Build history of the part. All positions in model axes, mm. Face numbers are marked on the shaded views. A direction names the side the tool comes from. Give positions to 0.01 mm unless a question says otherwise; leave off trailing zeros. Order: outer loops, then holes, each group sorted by start corner. A loop starts at its lowest first (then second) coordinate and runs counter-clockwise, first axis right, second up. Notation, with made-up numbers: M 31.5,-38 L 88.5,-38 A17 cw 88.5,-6 Z; hole C 9.5,55 d10. An arc over 180 degrees is marked long. Use CSV: the item, a comma, the result in double quotes. Start each with the question number.
Item 1: Wall check: line 1 along Z through (x, y) = (44, 17.75); line 2 along Z through (x, y) = (36.5, 1.25); line 3 along Y through (x, z) = (30.5, -3.5) (3 decimals). Give the ranges that are in metal, low to high.
Item 2: Band-saw the part on C-C on y = 22.5. Write the cut outline in (x, z), plus the area to 3 significant figures.
Item 3: Which spindle directions (+Z, -Z, +X, -X, +Y, -Y) get a long thin tool onto all of the face, cutting with end or side? Do the marked faces 1, 2 and 3. Say none if no direction does.
Item 4: Pin check, flat tips, straight feed: P1, Ø0.5, axis at x = 25, y = 1, coming from the -Z side; P2, Ø5, axis at x = 29, z = -4.5, coming from the -Y side (3 decimals); P3, Ø3, axis at x = 16.5, z = -2, coming from the +Y side (3 decimals); P4, Ø6, axis at y = 5.5, z = -3, coming from the -X side. Stop position of each tip, or through.
Item 5: Band-saw the part on B-B on z = -4. Write the cut outline in (x, y) (3 decimals), plus the area to 3 significant figures.
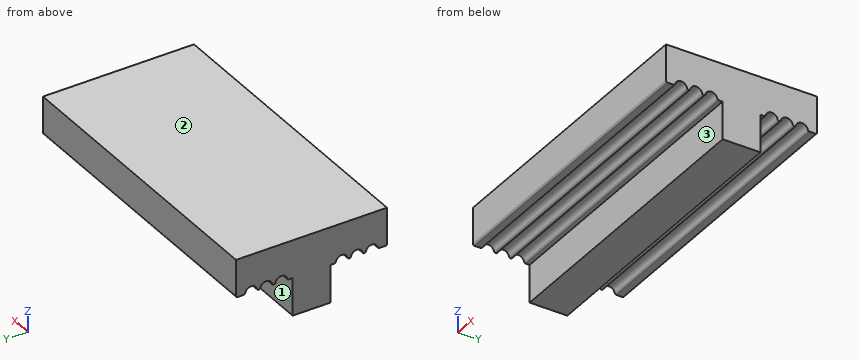
from build123d import *

# Parameters (mm, degrees)
F1_DEPTH = 50.8
F2_R     = 0.254


with BuildPart() as f1:
    # F0 (on Right) → F1 (new body)
    with BuildSketch(Plane.YZ):
        with BuildLine():
            Line((0, 6.35), (0, 0))
            Line((0, 0), (1.524, 0))
            ThreePointArc((1.524, 0), (2.54, 1.016), (3.556, 0))
            Line((3.556, 0), (4.064, 0))
            ThreePointArc((4.064, 0), (5.08, 1.016), (6.096, 0))
            Line((6.096, 0), (6.604, 0))
            ThreePointArc((6.604, 0), (7.62, 1.016), (8.636, 0))
            Line((8.636, 0), (9.525, 0))
            Line((9.525, 0), (9.525, -6.35))
            Line((9.525, -6.35), (15.875, -6.35))
            Line((15.875, -6.35), (15.875, 0))
            Line((15.875, 0), (16.764, 0))
            ThreePointArc((16.764, 0), (17.78, 1.016), (18.796, 0))
            Line((18.796, 0), (19.304, 0))
            ThreePointArc((19.304, 0), (20.32, 1.016), (21.336, 0))
            Line((21.336, 0), (21.844, 0))
            ThreePointArc((21.844, 0), (22.86, 1.016), (23.876, 0))
            Line((23.876, 0), (25.4, 0))
            Line((25.4, 0), (25.4, 6.35))
            Line((25.4, 6.35), (0, 6.35))
        make_face()
    extrude(amount=F1_DEPTH)

    # F2
    f2_edges = [f1.edges().sort_by_distance(p)[0] for p in [
        (25.4, 23.876, 0),
        (25.4, 25.4, 0),
        (25.4, 21.336, 0),
        (25.4, 18.796, 0),
        (25.4, 6.604, 0),
        (25.4, 4.064, 0),
        (25.4, 1.524, 0),
        (25.4, 0, 0),
        (25.4, 3.556, 0),
        (25.4, 6.096, 0),
        (25.4, 8.636, 0),
        (25.4, 16.764, 0),
        (25.4, 19.304, 0),
        (25.4, 21.844, 0),
    ]]
    fillet(f2_edges, radius=F2_R)


solid = f1.part
Model answer:
1,line 1,"z = 1.02 to 6.35"
1,line 2,"z = 0 to 6.35"
1,line 3,"y = 9.525 to 15.875"
2,outline,"M 0,0.95 L 50.8,0.95 L 50.8,6.35 L 0,6.35 Z"
2,area,"274 mm^2"
3,face 1,"-Z, +X, -X, +Y"
3,face 2,"+Z, +X, -X, +Y, -Y"
3,face 3,"-Z, +X, -X, -Y"
4,P1,"stops at z = 0"
4,P2,"stops at y = 9.525"
4,P3,"stops at y = 15.875"
4,P4,"passes through"
5,outline,"M 0,9.525 L 50.8,9.525 L 50.8,15.875 L 0,15.875 Z"
5,area,"323 mm^2"
